Here's how the part is built. I have some questions about the finished solid (model axes, mm). A direction names the side the tool comes from. Coordinates: 2 decimals unless noted, no trailing zeros. Write each loop counter-clockwise with the first axis right and the second up, starting at its lowest first coordinate (ties: lowest second). Pieces come first, ordered by that corner, then holes. Notation, with made-up numbers: M 78.25,87.25 L 92.25,87.25 A25 cw 92.25,125.25 Z; hole C 73,70 d3. An arc over 180 degrees is marked long. Use a Markdown table: item, result.
Autodesk Inventor part; units mm, degrees
ref_plane "YZ Plane" through (0, 0, 0) normal (1, 0, 0) x (0, 1, 0)
ref_plane "XZ Plane" through (0, 0, 0) normal (0, 1, 0) x (-1, 0, 0)
ref_plane "XY Plane" through (0, 0, 0) normal (0, 0, 1) x (1, 0, 0)
sketch "Boceto1" plane through (0, 0, 0) normal (0, 1, 0) x (-1, 0, 0)
  line L0 (-24.25, -40.9) -> (24.25, -40.9)
  line L1 (24.25, -40.9) -> (24.25, 40.9)
  line L2 (24.25, 40.9) -> (-24.25, 40.9)
  line L3 (-24.25, 40.9) -> (-24.25, -40.9)
  line L4 (-24.25, -40.9) -> (24.25, 40.9) construction
  line L5 (24.25, -40.9) -> (-24.25, 40.9) construction
  point P0 (0, 0)
  dimension "d0" = 48.5
  dimension "d1" = 81.8
extrude "Extrusión1" add sketch "Boceto1" along normal blind 1
sketch "Boceto2" plane through (0, 1, 0) normal (0, 1, 0) x (1, 0, 0)
  line L0 (3.1, 5.1) -> (-3.1, 5.1)
  line L1 (-3.1, 5.1) -> (-3.1, -5.1)
  line L2 (-3.1, -5.1) -> (3.1, -5.1)
  line L3 (3.1, -5.1) -> (3.1, 5.1)
  line L4 (3.1, 5.1) -> (-3.1, -5.1) construction
  line L5 (-3.1, 5.1) -> (3.1, -5.1) construction
  point P0 (0, 0)
  dimension "d4" = 6.2
  dimension "d5" = 10.2
extrude "Extrusión2" cut sketch "Boceto2" against normal blind 1
sketch "Boceto3" plane through (0, 0, 0) normal (0, -1, 0) x (1, 0, 0)
  line L0 (-22.25, -40.9) -> (-17.25, -40.9)
  line L1 (-17.25, -38.9) -> (-22.25, -38.9)
  line L2 (-17.25, -40.9) -> (-17.25, -38.9)
  line L3 (-22.25, 29.1) -> (-22.25, -40.9)
  line L4 (-22.25, 29.1) -> (-24.25, 29.1)
  line L5 (22.25, 38.9) -> (-24.25, 38.9)
  line L6 (-24.25, 29.1) -> (32.137, 29.1)
  line L7 (32.137, 29.1) -> (32.137, 38.9)
  line L8 (32.137, 38.9) -> (-24.25, 38.9)
  line L9 (-24.25, 38.9) -> (-24.25, 29.1)
  line L10 (-17.25, -40.9) -> (-22.25, -40.9)
  line L11 (-22.25, -40.9) -> (-22.25, -38.9)
  line L12 (-22.25, -38.9) -> (-17.25, -38.9)
  line L13 (-17.25, -38.9) -> (-17.25, -40.9)
  point P0 (0, 0)
extrude "Extrusión3" add sketch "Boceto3" along normal blind 4.3 contours L3 L1 L2 L0
sketch "Boceto4" plane through (0, 0, 0) normal (0, -1, 0) x (1, 0, 0)
  line L0 (-24.25, 29.1) -> (-22.25, 29.1)
  line L1 (-24.25, -40.9) -> (-24.25, 40.9)
  line L2 (-22.25, 29.1) -> (-24.25, 29.1)
  line L3 (-24.25, 29.1) -> (-24.25, 40.9)
  line L4 (-24.25, 40.9) -> (-22.25, 40.9)
  line L5 (-22.25, 40.9) -> (-22.25, 29.1)
  line L6 (-24.25, 38.9) -> (22.25, 38.9)
  point P0 (0, 0)
  point P1 (-22.25, 38.9)
extrude "Extrusión4" add sketch "Boceto4" along normal blind 8.85 contours L1 L6 L5 L0
sketch "Boceto5" plane through (0, 0, 0) normal (0, -1, 0) x (1, 0, 0)
  line L0 (24.25, -40.9) -> (24.25, 40.9)
  line L1 (24.25, 40.9) -> (-24.25, 40.9)
  line L2 (22.25, 38.9) -> (22.25, 29.1)
  line L3 (-24.25, 38.9) -> (22.25, 38.9)
  line L4 (22.25, 29.1) -> (-17.25, 29.1)
  line L5 (22.25, 38.9) -> (24.25, 38.9)
  line L6 (24.25, 38.9) -> (24.25, 29.1)
  line L7 (24.25, 29.1) -> (22.25, 29.1)
  line L8 (22.25, 29.1) -> (22.25, 38.9)
  point P0 (0, 0)
extrude "Extrusión5" add sketch "Boceto5" along normal blind 3.1
properties part number "TapaBaterias"
1. Suppose I cut it at C-C on y = -8. Write out the boundary of the cut face in (x, z), and give its area (3 significant figures).
Answers follow:
| item | result |
|---|---|
| outline | M -24.25,29.1 L -22.25,29.1 L -22.25,38.9 L -24.25,38.9 Z |
| area | 19.6 mm2 |
2. We'd pull the mould along X, two halves only. Please class faces 4 (the face through (24.25, 0.5, 9.3)), 5 (the face through (-22.25, -2, -40)), 6 (the face through (-20, -2, -38.9)), 7 (the face through (-22.25, -4, 34)): +X half, -X half, draft (parallel to the pull), parting line (faces both ways), or undercut.
Answers follow:
| item | result |
|---|---|
| face 4 | +X half |
| face 5 | -X half |
| face 6 | draft |
| face 7 | undercut |
3. Suppose I cut it at B-B on x = 15. Write out the boundary of the cut face in (y, z).
Answers follow:
| item | result |
|---|---|
| outline | M 0,-40.9 L 1,-40.9 L 1,40.9 L 0,40.9 Z |
4. Suppose I cut it at A-A on z = -2. Write out the boundary of the cut face in (x, y).
Answers follow:
| item | result |
|---|---|
| outline | M -24.25,0 L -3.1,0 L -3.1,1 L -24.25,1 Z; M 3.1,0 L 24.25,0 L 24.25,1 L 3.1,1 Z |
5. Will these pins go through, and if not, where does the flat tip stop? pin 1 Ø0.6 at (y, z) = (-1.5, -40) entering from +X; pin 2 Ø3.5 at (x, y) = (-19, -2.5) entering from +Z; pin 3 Ø2 at (y, z) = (-3, -40) entering from -X; pin 4 Ø3 at (y, z) = (-3, 0) entering from +X.
Answers follow:
| item | result |
|---|---|
| pin 1 | stops at x = -17.25 |
| pin 2 | stops at z = -38.9 |
| pin 3 | stops at x = -22.25 |
| pin 4 | passes through |
6. Which directions (+Z, -Z, +X, -X, +Y, -Y) give clear straight access to the entire face, cutting with the end or side of a thin tool? Please do faces 1 (the face through (-23, -4, 29.1)), 2 (the face through (-17.25, -2, -40)), 3 (the face through (23, -2, 38.9)).
Answers follow:
| item | result |
|---|---|
| face 1 | -Z, +X, -X, -Y |
| face 2 | +Z, -Z, +X, -Y |
| face 3 | +Z, +X, -X, -Y |
7. I need wall thicknesses on probe 1 along Y at (x, z) = (-7, -31.5); probe 2 along X at (y, z) = (-6, 38.5). Which ranges of each line are inside material? Lowest first, please.
Answers follow:
| item | result |
|---|---|
| probe 1 | y = 0 to 1 |
| probe 2 | x = -24.25 to -22.25 |
